```python
from build123d import *

# Parameters (mm, degrees)
SKETCH1_W           = 170
SKETCH1_H           = 340
BOSS_EXTRUDE1_DEPTH = 5
SKETCH2_R           = 2
CUT_EXTRUDE1_DEPTH  = 241.468293128
SKETCH3_R           = 2
SKETCH3_R_2         = 10.55
SKETCH3_R_3         = 1.5
BOSS_EXTRUDE2_DEPTH = 5
CHAMFER3_SIZE       = 5
FILLET1_R           = 10
CHAMFER2_SIZE       = 2
MIRROR2_OUTLINE_R   = 2
MIRROR2_OUTLINE_R_2 = 1.5
MIRROR2_OUTLINE_R_3 = 10.55
MIRROR2_DEPTH       = 5
SKETCH5_R           = 10.55
SKETCH5_R_2         = 2
BOSS_EXTRUDE3_DEPTH = 5
CHAMFER4_SIZE       = 2
FILLET2_R           = 10
SKETCH4_R           = 1.5
CUT_EXTRUDE2_DEPTH  = 325.221035715


# Read off the part's stored shape, not the designer's step: Mirror2
with BuildPart() as part:
    # Sketch1 → Boss-Extrude1 (new body)
    with BuildSketch(Plane.XY):
        with Locations((-85, 0)):
            Rectangle(SKETCH1_W, SKETCH1_H)
    extrude(amount=BOSS_EXTRUDE1_DEPTH)

    # Sketch2 → Cut-Extrude1 (cut, through all)
    with BuildSketch(Plane.XY.offset(5)):
        with Locations((-110, -160)):
            Circle(SKETCH2_R)
        with Locations((0, 160)):
            Circle(SKETCH2_R)
    extrude(amount=-CUT_EXTRUDE1_DEPTH, mode=Mode.SUBTRACT)

    # Sketch3 → Boss-Extrude2 (add)
    with BuildSketch(Plane.XY.offset(5)):
        with BuildLine():
            Line((-170, 170), (-143, 196.8))
            Line((-143, 196.8), (-143, 246.8))
            Line((-143, 246.8), (0, 246.8))
            Line((0, 246.8), (0, 239.85))
            ThreePointArc((0, 239.85), (-11.05, 228.8), (0, 217.75))
            Line((0, 217.75), (0, 170))
            Line((0, 170), (-170, 170))
        make_face()
        with Locations((-11.313708499, 240.113708499)):
            Circle(SKETCH3_R, mode=Mode.SUBTRACT)
        with Locations((-11.313708499, 217.486291501)):
            Circle(SKETCH3_R, mode=Mode.SUBTRACT)
        with Locations((-16, 228.8)):
            Circle(SKETCH3_R, mode=Mode.SUBTRACT)
        with Locations((-125, 228.8)):
            Circle(SKETCH3_R_2, mode=Mode.SUBTRACT)
        with Locations((-136.313708499, 240.113708499)):
            Circle(SKETCH3_R, mode=Mode.SUBTRACT)
        with Locations((-113.686291501, 240.113708499)):
            Circle(SKETCH3_R, mode=Mode.SUBTRACT)
        with Locations((-136.313708499, 217.486291501)):
            Circle(SKETCH3_R, mode=Mode.SUBTRACT)
        with Locations((-113.686291501, 217.486291501)):
            Circle(SKETCH3_R, mode=Mode.SUBTRACT)
        with Locations((-136.313708499, 198.8)):
            Circle(SKETCH3_R_3, mode=Mode.SUBTRACT)
    extrude(amount=-BOSS_EXTRUDE2_DEPTH)

    # Chamfer3
    chamfer3_edges = [part.edges().sort_by_distance(p)[0] for p in [
        (-170, -170, 2.5),
    ]]
    chamfer(chamfer3_edges, length=CHAMFER3_SIZE)

    # Fillet1
    fillet1_edges = [part.edges().sort_by_distance(p)[0] for p in [
        (-143, 196.8, 2.5),
        (-170, 170, 2.5),
    ]]
    fillet(fillet1_edges, radius=FILLET1_R)

    # Chamfer2
    chamfer2_edges = [part.edges().sort_by_distance(p)[0] for p in [
        (-143, 246.8, 2.5),
    ]]
    chamfer(chamfer2_edges, length=CHAMFER2_SIZE)

    # Mirror2 outline → Mirror2 (add)
    with BuildSketch(Plane.XY):
        with BuildLine():
            Line((0, -170), (165, -170))
            Line((165, -170), (170, -165))
            Line((170, -165), (170, 165.836071225))
            ThreePointArc((170, 165.836071225), (169.231666328, 169.680071331), (167.044732637, 172.933376494))
            Line((167.044732637, 172.933376494), (145.955267363, 193.866623506))
            ThreePointArc((145.955267363, 193.866623506), (143.768333672, 197.119928669), (143, 200.963928775))
            Line((143, 200.963928775), (143, 244.8))
            Line((143, 244.8), (141, 246.8))
            Line((141, 246.8), (0, 246.8))
            Line((0, 246.8), (0, 239.85))
            ThreePointArc((0, 239.85), (11.05, 228.8), (0, 217.75))
            Line((0, 217.75), (0, 162))
            ThreePointArc((0, 162), (2, 160), (0, 158))
            Line((0, 158), (0, -170))
        make_face()
        with Locations((110, -160)):
            Circle(MIRROR2_OUTLINE_R, mode=Mode.SUBTRACT)
        with Locations((11.313708499, 217.486291501)):
            Circle(MIRROR2_OUTLINE_R, mode=Mode.SUBTRACT)
        with Locations((11.313708499, 240.113708499)):
            Circle(MIRROR2_OUTLINE_R, mode=Mode.SUBTRACT)
        with Locations((16, 228.8)):
            Circle(MIRROR2_OUTLINE_R, mode=Mode.SUBTRACT)
        with Locations((113.686291501, 217.486291501)):
            Circle(MIRROR2_OUTLINE_R, mode=Mode.SUBTRACT)
        with Locations((113.686291501, 240.113708499)):
            Circle(MIRROR2_OUTLINE_R, mode=Mode.SUBTRACT)
        with Locations((136.313708499, 198.8)):
            Circle(MIRROR2_OUTLINE_R_2, mode=Mode.SUBTRACT)
        with Locations((136.313708499, 217.486291501)):
            Circle(MIRROR2_OUTLINE_R, mode=Mode.SUBTRACT)
        with Locations((125, 228.8)):
            Circle(MIRROR2_OUTLINE_R_3, mode=Mode.SUBTRACT)
        with Locations((136.313708499, 240.113708499)):
            Circle(MIRROR2_OUTLINE_R, mode=Mode.SUBTRACT)
    extrude(amount=MIRROR2_DEPTH)

    # Sketch5 → Boss-Extrude3 (add)
    # profile 1 of 2: a face of its own
    with BuildSketch(Plane.XY.offset(5)):
        Polygon((-198.9, -163.26), (-198.9, -197.26), (-164.9, -197.26), (-117.684294986, -170), (-170, -113.203731661), align=None)
        with Locations((-182.9, -181.26)):
            Circle(SKETCH5_R, mode=Mode.SUBTRACT)
        with Locations((-194.213708499, -169.946291501)):
            Circle(SKETCH5_R_2, mode=Mode.SUBTRACT)
        with Locations((-171.586291501, -169.946291501)):
            Circle(SKETCH5_R_2, mode=Mode.SUBTRACT)
        with Locations((-171.586291501, -192.573708499)):
            Circle(SKETCH5_R_2, mode=Mode.SUBTRACT)
        with Locations((-194.213708499, -192.573708499)):
            Circle(SKETCH5_R_2, mode=Mode.SUBTRACT)
    # profile 2 of 2: a face of its own
    with BuildSketch(Plane.XY.offset(5)):
        Polygon((176.2, -197.26), (210.2, -197.26), (210.2, -163.26), (170, -93.631557536), (128.984294986, -170), align=None)
        with Locations((194.2, -181.26)):
            Circle(SKETCH5_R, mode=Mode.SUBTRACT)
        with Locations((205.513708499, -192.573708499)):
            Circle(SKETCH5_R_2, mode=Mode.SUBTRACT)
        with Locations((205.513708499, -169.946291501)):
            Circle(SKETCH5_R_2, mode=Mode.SUBTRACT)
        with Locations((182.886291501, -169.946291501)):
            Circle(SKETCH5_R_2, mode=Mode.SUBTRACT)
        with Locations((182.886291501, -192.573708499)):
            Circle(SKETCH5_R_2, mode=Mode.SUBTRACT)
    extrude(amount=-BOSS_EXTRUDE3_DEPTH)

    # Chamfer4
    chamfer4_edges = [part.edges().sort_by_distance(p)[0] for p in [
        (-198.9, -197.26, 2.5),
        (210.2, -197.26, 2.5),
    ]]
    chamfer(chamfer4_edges, length=CHAMFER4_SIZE)

    # Fillet2
    fillet2_edges = [part.edges().sort_by_distance(p)[0] for p in [
        (-198.9, -163.26, 2.5),
        (-170, -113.203731661, 2.5),
        (-117.684294986, -170, 2.5),
        (-164.9, -197.26, 2.5),
        (176.2, -197.26, 2.5),
        (128.984294986, -170, 2.5),
        (170, -93.631557536, 2.5),
        (210.2, -163.26, 2.5),
    ]]
    fillet(fillet2_edges, radius=FILLET2_R)

    # Sketch4 → Cut-Extrude2 (cut, through all)
    with BuildSketch(Plane.XY.offset(5)):
        with Locations((-85, 160)):
            Circle(SKETCH4_R)
        with Locations((-85, 130)):
            Circle(SKETCH4_R)
        with Locations((-85, 100)):
            Circle(SKETCH4_R)
        with Locations((-85, 70)):
            Circle(SKETCH4_R)
        with Locations((-85, 40)):
            Circle(SKETCH4_R)
        with Locations((-85, 10)):
            Circle(SKETCH4_R)
        with Locations((-85, -20)):
            Circle(SKETCH4_R)
        with Locations((-85, -50)):
            Circle(SKETCH4_R)
        with Locations((-85, -80)):
            Circle(SKETCH4_R)
        with Locations((-85, -110)):
            Circle(SKETCH4_R)
    cut_extrude2 = extrude(amount=-CUT_EXTRUDE2_DEPTH, mode=Mode.SUBTRACT)

    # Mirror3: Cut-Extrude2 across plane
    add(cut_extrude2.mirror(Plane(origin=(0, 0, 0), x_dir=(0, 0, 1), z_dir=(1, 0, 0))), mode=Mode.SUBTRACT)


solid = part.part
```
Input: part model. Units: mm. Frame: model coordinates. A direction names the side the tool comes from. Give positions to 0.01 mm unless a question says otherwise; leave off trailing zeros. Order: outer loops, then holes, each group sorted by start corner. A loop starts at its lowest first (then second) coordinate and runs counter-clockwise, first axis right, second up.
1. Section C-C on x = 48. Return the cut outline in (y, z).
Derived:
outline: (-170, 0) - (246.8, 0) - (246.8, 5) - (-170, 5) - close
2. Section D-D on z = 1.15. Give the number of separate pieces and of enclosed holes in the cut face, and give its area (3 significant figures).
Derived:
separate pieces: 1
enclosed holes: 52
area: 142,000 mm2
3. Reachability of faces 4 (the flat face through (-184.266, -137.914, 2.535)), 5 (the flat face through (152.294, -183.458, 2.535)) from +Z, -Z, +X, -X, +Y, -Y: full face, straight path, thin tool, end or side. Return the list, or none.
Derived:
face 4: +Z, -Z, -X, +Y
face 5: +Z, -Z, -Y
4. Material intervals for L1, parallel to X at y = 160, z = 3.2; L2, parallel to Y at x = -114, z = 1.15; L3, parallel to Y at x = 16, z = 2.95, sorted ascending.
Derived:
L1: x = -170 to -86.5, -83.5 to -2, 2 to 83.5, 86.5 to 170
L2: y = -170 to 215.51, 219.46 to 238.14, 242.09 to 246.8
L3: y = -170 to 226.8, 230.8 to 246.8
5. Section A-A on x = 194.2. Return the cut outline in (y, z).
Derived:
outline: (-197.26, 0) - (-191.81, 0) - (-191.81, 5) - (-197.26, 5) - close; (-170.71, 0) - (-135.55, 0) - (-135.55, 5) - (-170.71, 5) - close
6. Pin query (flat end, axial travel): pin 1 (2.5 mm diameter, centred on y = 81.5, z = 3, fed in from +X); pin 2 (1.5 mm diameter, centred on x = 49, z = 4.5, fed in from -Y). Return the tip coordinate at first contact, or that it passes through.
Derived:
pin 1: stops at x = 170
pin 2: stops at y = -170
7. Section B-B on y = -66. Return the cut outline in (x, z).
Derived:
outline: (-170, 0) - (170, 0) - (170, 5) - (-170, 5) - close
8. Mould query, pull axis X, two halves, no side actions, for faces 1 (the flat face through (-156.6, 183.3, 2.5)), 2 (the flat face through (3, 28, 0)), 3 (the flat face through (-141.59, -183.8, 2.54)). Classes: released by +X, released by -X, zero draft, split by the parting line, or undercut.
Derived:
face 1: released by -X
face 2: zero draft
face 3: undercut
